Check sheet for the modelled part. Datum: model origin and axes. Units: mm. Face numbers are marked on the shaded views. A direction names the side the tool comes from. Coordinates: 2 decimals unless noted, no trailing zeros. Loops run counter-clockwise (first coordinate to the right, second up) from the corner with the lowest first, then second, coordinate; pieces in that order, holes last.
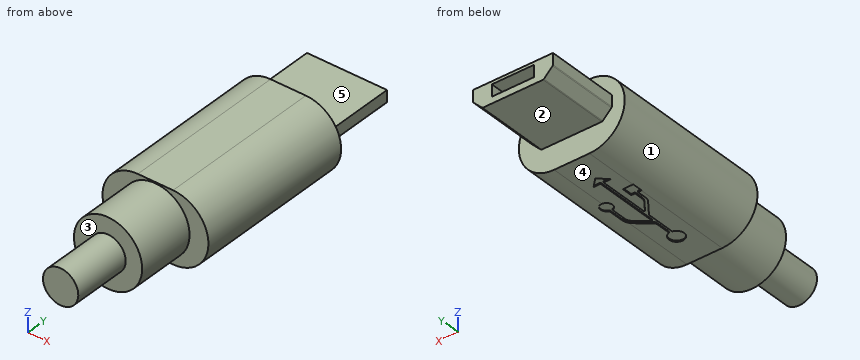
```python
from build123d import *

# Parameters (mm, degrees)
EXTRUDE_1_DEPTH     = 14
SKETCH_2_R          = 2.9
EXTRUDE_2_DEPTH     = 5
EXTRUDE_3_DEPTH     = 6.2
SKETCH_5_W          = 3.6
SKETCH_5_H          = 1
CUT_EXTRUDE_1_DEPTH = 4
FILLET_1_R          = 0.1
SKETCH_6_R          = 1.5
EXTRUDE_4_DEPTH     = 5
CUT_EXTRUDE_2_DEPTH = 0.1


with BuildPart() as part:
    # 草图1 → 凸台-拉伸1 (new body)
    with BuildSketch(Plane(origin=(0, 0, 0), x_dir=(1, 0, 0), z_dir=(0, 1, 0))):
        with BuildLine():
            Line((-1.5, 3), (1.5, 3))
            ThreePointArc((1.5, 3), (4.5, 0), (1.5, -3))
            Line((1.5, -3), (-1.5, -3))
            ThreePointArc((-1.5, -3), (-4.5, 0), (-1.5, 3))
        make_face()
    extrude(amount=EXTRUDE_1_DEPTH)

    # 草图2 → 凸台-拉伸2 (add)
    with BuildSketch(Plane.XZ):
        with Locations(Location((0, 0, 0), (0, 0, 270))):
            Circle(SKETCH_2_R)
    extrude(amount=EXTRUDE_2_DEPTH)

    # 草图3 → 凸台-拉伸3 (add)
    with BuildSketch(Plane(origin=(0, 14, 0), x_dir=(1, 0, 0), z_dir=(0, 1, 0))):
        Polygon((-3.4, 0.1), (-2.6, 0.9), (2.6, 0.9), (3.4, 0.1), (3.4, -0.9), (-3.4, -0.9), align=None)
    extrude(amount=EXTRUDE_3_DEPTH)

    # 草图5 → 切除-拉伸1 (cut)
    with BuildSketch(Plane(origin=(0, 20.2, 0), x_dir=(1, 0, 0), z_dir=(0, 1, 0))):
        with Locations((0, -0.15)):
            Rectangle(SKETCH_5_W, SKETCH_5_H)
    extrude(amount=-CUT_EXTRUDE_1_DEPTH, mode=Mode.SUBTRACT)

    # 圆角1
    fillet_1_edges = [part.edges().sort_by_distance(p)[0] for p in [
        (3.4, 17.1, -0.1),
        (2.6, 17.1, -0.9),
        (-2.6, 17.1, -0.9),
        (-3.4, 17.1, -0.1),
    ]]
    fillet(fillet_1_edges, radius=FILLET_1_R)

    # 草图6 → 凸台-拉伸4 (add)
    with BuildSketch(Plane.XZ.offset(5)):
        with Locations(Location((0, 0, 0), (0, 0, 270))):
            Circle(SKETCH_6_R)
    extrude(amount=EXTRUDE_4_DEPTH)

    # 草图8 → 切除-拉伸2 (cut)
    with BuildSketch(Plane(origin=(0, 0, -3), x_dir=(-1, 0, 0), z_dir=(0, 0, -1))):
        with BuildLine():
            Line((0, 11.52960021), (-0.716956191, 10.8097184))
            Line((-0.716956191, 10.8097184), (-0.127, 10.8097184))
            Line((-0.127, 10.8097184), (-0.127, 5.401898496))
            ThreePointArc((-0.127, 5.401898496), (-0.156162493, 5.355937009), (-0.21016765, 5.362745269))
            Line((-0.21016765, 5.362745269), (-1.120514747, 6.115321688))
            ThreePointArc((-1.120514747, 6.115321688), (-1.324422308, 6.378057505), (-1.397, 6.702620106))
            Line((-1.397, 6.702620106), (-1.397, 7.963089706))
            ThreePointArc((-1.397, 7.963089706), (-1.524, 8.962958591), (-1.651, 7.963089706))
            Line((-1.651, 7.963089706), (-1.651, 6.722530894))
            ThreePointArc((-1.651, 6.722530894), (-1.550201428, 6.271766401), (-1.267007097, 5.906869222))
            Line((-1.267007097, 5.906869222), (-0.219161751, 5.040624136))
            ThreePointArc((-0.219161751, 5.040624136), (-0.151192564, 4.953045531), (-0.127, 4.844857997))
            Line((-0.127, 4.844857997), (-0.127, 3.56953501))
            ThreePointArc((-0.127, 3.56953501), (0, 2.312364615), (0.127, 3.56953501))
            Line((0.127, 3.56953501), (0.127, 5.933535284))
            ThreePointArc((0.127, 5.933535284), (0.139930568, 6.013544838), (0.177405738, 6.08540818))
            Line((0.177405738, 6.08540818), (1.053118903, 7.259351528))
            ThreePointArc((1.053118903, 7.259351528), (1.165544414, 7.474941553), (1.204336117, 7.714970215))
            Line((1.204336117, 7.714970215), (1.204336117, 8.518458591))
            Line((1.204336117, 8.518458591), (1.524, 8.518458591))
            Line((1.524, 8.518458591), (1.524, 9.407458591))
            Line((1.524, 9.407458591), (0.635, 9.407458591))
            Line((0.635, 9.407458591), (0.635, 8.518458591))
            Line((0.635, 8.518458591), (0.954663883, 8.518458591))
            Line((0.954663883, 8.518458591), (0.954663883, 7.798383163))
            ThreePointArc((0.954663883, 7.798383163), (0.915872181, 7.558354501), (0.80344667, 7.342764476))
            Line((0.80344667, 7.342764476), (0.218518852, 6.558635439))
            ThreePointArc((0.218518852, 6.558635439), (0.161798089, 6.540796132), (0.127, 6.589010019))
            Line((0.127, 6.589010019), (0.127, 10.8097184))
            Line((0.127, 10.8097184), (0.716956191, 10.8097184))
            Line((0.716956191, 10.8097184), (0, 11.52960021))
        make_face()
    extrude(amount=-CUT_EXTRUDE_2_DEPTH, mode=Mode.SUBTRACT)


solid = part.part
```
1) Set-up check for the marked faces 1, 2, 3, 4 and 5: record each of +Z, -Z, +X, -X, +Y, -Y from which the full face is reachable in a straight line by a thin tool's end or side.
Answer sheet:
face 1: -X, +Y, -Y
face 2: -Z, +X, -X, +Y
face 3: -Y
face 4: -Z, +X, -X, +Y, -Y
face 5: +Z, +X, -X, +Y
2) Section check A-A on y = 4. Enter the section's corners in (x, z), plus the area to 3 significant figures.
Answer sheet:
outline: (-1.5, -3) - (-0.13, -3) - (-0.13, -2.9) - (0.13, -2.9) - (0.13, -3) - (1.5, -3) arc R3 ccw to (1.5, 3) - (-1.5, 3) arc R3 ccw to start
area: 46.2 mm2
3) Section check B-B on y = -3. Enter the section's corners in (x, z).
Answer sheet:
outline: circle Ø5.8 at (0, 0)
4) Scan lines: line 1 (Y direction, x = -1, z = -1.25); line 2 (X direction, y = 18.5, z = 0.25); line 3 (Z direction, x = 1.25, y = 17). Record each from-to range of solid material in increasing order.
Answer sheet:
line 1: y = -5 to 14
line 2: x = -3.4 to -1.8, 1.8 to 3.4
line 3: z = -0.9 to -0.35, 0.65 to 0.9
5) Depth check by flat-ended pin: pin 1 (0.8 mm diameter, centred on y = 18, z = 0.5, fed in from -X); pin 2 (1.5 mm diameter, centred on x = 0, y = 18.5, fed in from -Z); pin 3 (5 mm diameter, centred on x = 2.5, y = -6, fed in from +Z). Enter the tip coordinate at first touch or a pass-through.
Answer sheet:
pin 1: stops at x = -3.4
pin 2: stops at z = -0.9
pin 3: stops at z = 2.89
